Design review of the part built by this model. Coordinates are the model's own, in mm. Face numbers are marked on the shaded views. Give positions to 0.01 mm unless a question says otherwise; leave off trailing zeros. Order: outer loops, then holes, each group sorted by start corner. A loop starts at its lowest first (then second) coordinate and runs counter-clockwise, first axis right, second up.
```python
from build123d import *

# Parameters (mm, degrees)
SKETCH2_R          = 12.7
CUT_EXTRUDE1_DEPTH = 67.514107143


with BuildPart() as part:
    # Sketch1 → Revolve1 (revolve)
    with BuildSketch(Plane.XY, mode=Mode.PRIVATE) as revolve1_sk:
        Polygon((0, -77.674107143), (-127, -77.674107143), (-127, -64.974107143), (-83.230357143, -64.974107143), (-83.230357143, -14.174107143), (-83.230357143, 62.025892857), (-75.610357143, 62.025892857), (-75.610357143, 74.725892857), (-83.230357143, 74.725892857), (-83.230357143, 100.125892857), (-72.117857143, 100.125892857), (-72.117857143, 138.225892857), (-59.417857143, 138.225892857), (-59.417857143, -64.974107143), (0, -64.974107143), align=None)
    revolve(revolve1_sk.sketch.rotate(Axis((0, 71.324107143, 0), (0, -1, 0)), 270), axis=Axis((0, 71.324107143, 0), (0, -1, 0)))

    # Sketch2 → Cut-Extrude1 (cut)
    with BuildSketch(Plane(origin=(0, 0, 0), x_dir=(1, 0, 0), z_dir=(0, 1, 0))):
        with Locations(Location((-102.608331848, 0, 0), (0, 0, 270))):
            Circle(SKETCH2_R)
        with Locations(Location((0, -105.234824984, 0), (0, 0, 270))):
            Circle(SKETCH2_R)
        with Locations(Location((102.258132763, 0, 0), (0, 0, 270))):
            Circle(SKETCH2_R)
        with Locations(Location((0, 99.281440542, 0), (0, 0, 270))):
            Circle(SKETCH2_R)
    extrude(amount=-CUT_EXTRUDE1_DEPTH, mode=Mode.SUBTRACT)


solid = part.part
```
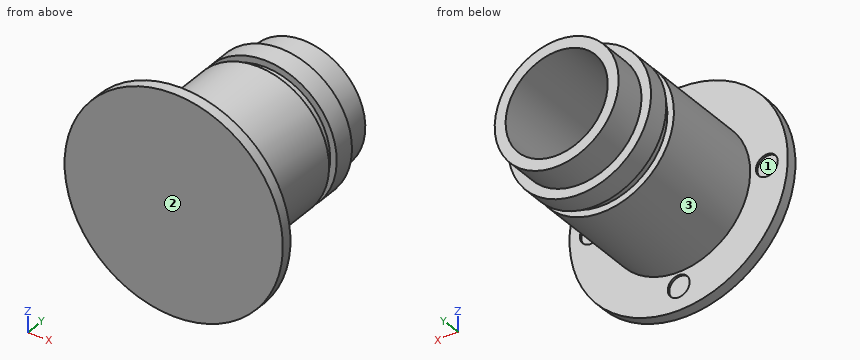
1. For line 1 along X through (y, z) = (-66.7, 0); line 2 along Y through (x, z) = (63.5, -46); line 3 along X through (y, z) = (38.5, 0), list the stretches that pass through material, from the lowest coordinate up.
Recorded:
line 1: x = -127 to -115.31, -89.91 to 89.56, 114.96 to 127
line 2: y = -77.67 to 62.03, 74.73 to 100.13
line 3: x = -83.23 to -59.42, 59.42 to 83.23
2. Take a section at B-B (z = -38.5). State the section outline as (x, y) points.
Recorded:
outline: (-121.02, -77.67) - (121.02, -77.67) - (121.02, -64.97) - (73.79, -64.97) - (73.79, 62.03) - (65.07, 62.03) - (65.07, 74.73) - (73.79, 74.73) - (73.79, 100.13) - (60.98, 100.13) - (60.98, 138.23) - (45.26, 138.23) - (45.26, -64.97) - (-45.26, -64.97) - (-45.26, 138.23) - (-60.98, 138.23) - (-60.98, 100.13) - (-73.79, 100.13) - (-73.79, 74.73) - (-65.07, 74.73) - (-65.07, 62.03) - (-73.79, 62.03) - (-73.79, -64.97) - (-121.02, -64.97) - close
3. For pin 1 (3 mm diameter, centred on x = -64, y = 34.5, fed in from -Z); pin 2 (10 mm diameter, centred on y = -19.5, z = 27.5, fed in from -X); pin 3 (1 mm diameter, centred on x = 68.5, y = -53.5, fed in from -Z), all flat-tipped, find the tip position at first contact; note any pin that passes through.
Recorded:
pin 1: stops at z = -54.96
pin 2: stops at x = -80.13
pin 3: stops at z = -47.99
4. Take a section at C-C (y = -4.5). State the section outline as (x, z) points, then the cut area to 3 significant figures.
Recorded:
outline: circle Ø166.46 at (0, 0); hole circle Ø118.84 at (0, 0)
area: 10,700 mm2
5. Take a section at D-D (x = -79.5). State the section outline as (y, z) points, then the cut area to 3 significant figures.
Recorded:
outline: (-77.67, -99.04) - (-64.97, -99.04) - (-64.97, -24.64) - (62.03, -24.64) - (62.03, 24.64) - (-64.97, 24.64) - (-64.97, 99.04) - (-77.67, 99.04) - close; (74.73, -24.64) - (100.13, -24.64) - (100.13, 24.64) - (74.73, 24.64) - close
area: 10,000 mm2
6. Draft analysis for pull direction X (two halves, no side actions). For the marked faces 1, 2 and 3, state which applies: pulls with the +X half, pulls with the -X half, needs draft (parallel to the pull), parting line crosses it, or undercut.
Recorded:
face 1: undercut
face 2: needs draft
face 3: parting line crosses it
